from build123d import *

# Parameters (mm, degrees)
F1_DEPTH  = 17.3
F3_DEPTH  = 11.501
F5_DEPTH  = 3
F8_DEPTH  = 10.501
F9_W      = 3
F9_H      = 9.6
F9_H_2    = 1
F10_DEPTH = 10


with BuildPart() as f1:
    # F0 (on Front) → F1 (new body)
    with BuildSketch(Plane.XZ):
        with BuildLine():
            Line((6.5, 11.5), (0, 11.5))
            Line((0, 11.5), (-6.5, 11.5))
            ThreePointArc((-6.5, 11.5), (-7.207107, 11.207107), (-7.5, 10.5))
            Line((-7.5, 10.5), (-7.5, 6))
            ThreePointArc((-7.5, 6), (-8.37868, 3.87868), (-10.5, 3))
            Line((-10.5, 3), (-13.3, 3))
            Line((-13.3, 3), (-13.3, 0))
            Line((-13.3, 0), (-6, 0))
            Line((-6, 0), (-6, 7))
            ThreePointArc((-6, 7), (-5.12132, 9.12132), (-3, 10))
            Line((-3, 10), (0, 10))
            Line((0, 10), (3, 10))
            ThreePointArc((3, 10), (5.12132, 9.12132), (6, 7))
            Line((6, 7), (6, 0))
            Line((6, 0), (13.3, 0))
            Line((13.3, 0), (13.3, 3))
            Line((13.3, 3), (10.5, 3))
            ThreePointArc((10.5, 3), (8.37868, 3.87868), (7.5, 6))
            Line((7.5, 6), (7.5, 10.5))
            ThreePointArc((7.5, 10.5), (7.207107, 11.207107), (6.5, 11.5))
        make_face()
    extrude(amount=F1_DEPTH)

    # F2 (on face) → F3 (intersect, through all)
    with BuildSketch(Plane.XY.offset(11.5)):
        with BuildLine():
            Line((6.5, 0), (-6.5, 0))
            Line((-6.5, 0), (-7.5, 0))
            Line((-7.5, 0), (-9.05, 0))
            ThreePointArc((-9.05, 0), (-12.055204, -1.244796), (-13.3, -4.25))
            ThreePointArc((-13.3, -4.25), (-12.055204, -7.255204), (-9.05, -8.5))
            Line((-9.05, -8.5), (-7.5, -8.5))
            Line((-7.5, -8.5), (-7.5, -17.3))
            Line((-7.5, -17.3), (-6.5, -17.3))
            Line((-6.5, -17.3), (6.5, -17.3))
            Line((6.5, -17.3), (7.5, -17.3))
            Line((7.5, -17.3), (7.5, -8.5))
            Line((7.5, -8.5), (9.05, -8.5))
            ThreePointArc((9.05, -8.5), (12.055204, -7.255204), (13.3, -4.25))
            ThreePointArc((13.3, -4.25), (12.055204, -1.244796), (9.05, 0))
            Line((9.05, 0), (7.5, 0))
            Line((7.5, 0), (6.5, 0))
        make_face()
    extrude(amount=-F3_DEPTH, mode=Mode.INTERSECT)

    # F4 (on face) → F5 (cut)
    with BuildSketch(Plane(origin=(0, 0, 0), x_dir=(1, 0, 0), z_dir=(0, 0, -1))):
        with BuildLine():
            Line((-7.5, 6.25), (-7.5, 5.5))
            Line((-7.5, 5.5), (-9.05, 5.5))
            ThreePointArc((-9.05, 5.5), (-10.3, 4.25), (-9.05, 3))
            Line((-9.05, 3), (-7.5, 3))
            Line((-7.5, 3), (-7.5, 2.25))
            Line((-7.5, 2.25), (-6, 2.25))
            Line((-6, 2.25), (-6, 6.25))
            Line((-6, 6.25), (-7.5, 6.25))
        make_face()
        with BuildLine():
            Line((7.5, 6.25), (6, 6.25))
            Line((6, 6.25), (6, 2.25))
            Line((6, 2.25), (7.5, 2.25))
            Line((7.5, 2.25), (7.5, 3))
            Line((7.5, 3), (9.05, 3))
            ThreePointArc((9.05, 3), (10.3, 4.25), (9.05, 5.5))
            Line((9.05, 5.5), (7.5, 5.5))
            Line((7.5, 5.5), (7.5, 6.25))
        make_face()
    extrude(amount=-F5_DEPTH, mode=Mode.SUBTRACT)

    # F7 (on offset) → F8 (cut, through all)
    with BuildSketch(Plane.XY.offset(1)):
        Polygon((-11.648076, -2.75), (-11.648076, -5.75), (-9.05, -7.25), (-7.5, -6.355107), (-7.5, -2.144893), (-9.05, -1.25), align=None)
        Polygon((7.5, -2.144893), (7.5, -6.355107), (9.05, -7.25), (11.648076, -5.75), (11.648076, -2.75), (9.05, -1.25), align=None)
    extrude(amount=F8_DEPTH, mode=Mode.SUBTRACT)

    # F9 (on face) → F10 (cut, through all)
    with BuildSketch(Plane(origin=(0, 0, 0), x_dir=(1, 0, 0), z_dir=(0, 0, -1))):
        with Locations((-4.5, 12.5)):
            Rectangle(F9_W, F9_H)
        with Locations((4.5, 16.8)):
            Rectangle(F9_W, F9_H_2)
        with Locations((4.5, 8.2)):
            Rectangle(F9_W, F9_H_2)
        with Locations((4.5, 11.2)):
            Rectangle(F9_W, F9_H_2)
    extrude(amount=-F10_DEPTH, mode=Mode.SUBTRACT)


solid = f1.part
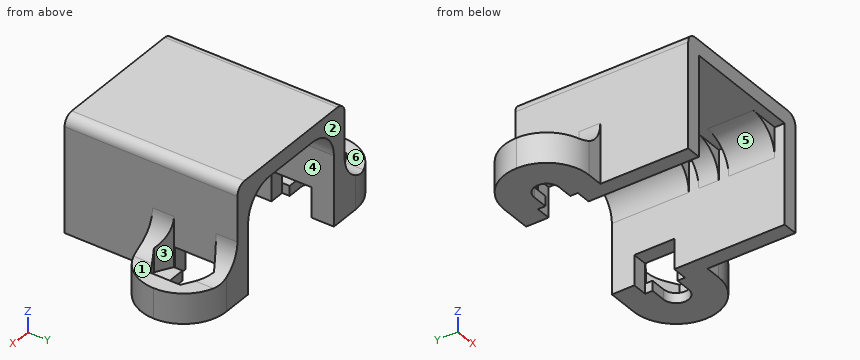
Can you work these out from the model? Positions are in its coordinate system, mm. Face numbers are marked on the shaded views. A direction names the side the tool comes from. Give positions to 0.01 mm unless a question says otherwise; leave off trailing zeros. Loops run counter-clockwise (first coordinate to the right, second up) from the corner with the lowest first, then second, coordinate; pieces in that order, holes last. Notation, with made-up numbers: (4.25, 35.5) -> (57.25, 35.5) arc R19 ccw to (57.25, 65.5) -> close; hole circle Ø3 at (74.25, -1.5). An arc over 180 degrees is marked (long way). Return JSON: item names as keys, results as strings.
Q1. We'd pull the mould along Y, two halves only. Please class the marked faces 1, 2 and 3: released by +Y, released by -Y, zero draft, split by the parting line, or undercut.
Checks:
{"face 1": "zero draft", "face 2": "released by +Y", "face 3": "undercut"}
Q2. I want a section at C-C, the plane x = -11.25. List the corners of the cut face in (y, z) for me.
Checks:
{"outline": "(-7.89, 0) -> (-0.61, 0) -> (-0.61, 3) -> (-2.52, 3) -> (-2.52, 1) -> (-5.98, 1) -> (-5.98, 3) -> (-7.89, 3) -> close"}
Q3. I want a section at B-B, the plane y = -3.75. List the corners of the cut face in (x, z) for me, then the cut area to 3 significant figures.
Checks:
{"outline": "(-13.27, 0) -> (-10.2, 0) -> (-10.2, 1) -> (-11.65, 1) -> (-11.65, 3) -> (-13.27, 3) -> close; (-7.5, 3) -> (-6, 3) -> (-6, 7) arc R3 cw to (-3, 10) -> (3, 10) arc R3 cw to (6, 7) -> (6, 3) -> (7.5, 3) -> (7.5, 10.5) arc R1 ccw to (6.5, 11.5) -> (-6.5, 11.5) arc R1 ccw to (-7.5, 10.5) -> close; (10.2, 0) -> (13.27, 0) -> (13.27, 3) -> (11.65, 3) -> (11.65, 1) -> (10.2, 1) -> close", "area": "59.6 mm2"}
Q4. On a 3-axis mill with a long thin cutter (end or side, diameter ignored), from which of +Z, -Z, +X, -X, +Y, -Y can I reach the whole of each face in a straight line? I mean the marked faces 4, 5 and 6. Say none if no direction works.
Checks:
{"face 4": "-Z, -Y", "face 5": "-Z, +Y, -Y", "face 6": "+Z, -X, +Y, -Y"}
Q5. For pin 1 Ø3 at (y, z) = (-9, 7.5) entering from +X; pin 2 Ø5 at (y, z) = (-7.5, 7.5) entering from -X; pin 3 Ø0.8 at (y, z) = (-6, 0.5) entering from -X; pin 4 Ø0.9 at (x, z) = (4, 8.5) entering from -Y, each with a flat end and sliding along its axis, tell me the tip position at first contact or that it passes through.
Checks:
{"pin 1": "stops at x = 7.5", "pin 2": "stops at x = -7.67", "pin 3": "stops at x = -13.08", "pin 4": "passes through"}
Q6. I want a section at D-D, the plane z = 9.5. List the corners of the cut face in (x, y) for me, then the cut area to 3 significant figures.
Checks:
{"outline": "(-7.5, -17.3) -> (-6, -17.3) -> (-6, -7.7) -> (-4.66, -7.7) -> (-4.66, 0) -> (-7.5, 0) -> close; (4.66, -16.3) -> (6, -16.3) -> (6, -17.3) -> (7.5, -17.3) -> (7.5, 0) -> (4.66, 0) -> (4.66, -7.7) -> (6, -7.7) -> (6, -8.7) -> (4.66, -8.7) -> (4.66, -10.7) -> (6, -10.7) -> (6, -11.7) -> (4.66, -11.7) -> close", "area": "81.4 mm2"}
Q7. I need wall thicknesses on probe 1 along X at (y, z) = (-10.25, 0.5); probe 2 along Z at (x, y) = (2.5, -14); probe 3 along X at (y, z) = (-12.75, 9). Which ranges of each line are inside material? Lowest first, please.
Checks:
{"probe 1": "x = -7.5 to -6, 6 to 7.5", "probe 2": "z = 10 to 11.5", "probe 3": "x = -7.5 to -6, 5.24 to 7.5"}
